from build123d import *

# Parameters (mm, degrees)
SALIENTE_EXTRUIR1_DEPTH = 10
CROQUIS2_R              = 3.5
SALIENTE_EXTRUIR2_DEPTH = 11
CROQUIS3_R              = 1
CORTAR_EXTRUIR1_DEPTH   = 40


with BuildPart() as part:
    # Croquis1 → Saliente-Extruir1 (new body)
    with BuildSketch(Plane(origin=(0, 0, 0), x_dir=(1, 0, 0), z_dir=(0, 1, 0))):
        Polygon((0, 6.639528096), (-5.75, 3.319764048), (-5.75, -3.319764048), (0, -6.639528096), (5.75, -3.319764048), (5.75, 3.319764048), align=None)
    extrude(amount=SALIENTE_EXTRUIR1_DEPTH)

    # Croquis2 → Saliente-Extruir2 (add)
    with BuildSketch(Plane.XZ):
        with Locations(Location((0, 0, 0), (0, 0, 270))):
            Circle(CROQUIS2_R)
    extrude(amount=SALIENTE_EXTRUIR2_DEPTH)

    # Croquis3 → Cortar-Extruir1 (cut)
    with BuildSketch(Plane.XZ.offset(11)):
        with Locations(Location((0, 0, 0), (0, 0, 270))):
            Circle(CROQUIS3_R)
    extrude(amount=-CORTAR_EXTRUIR1_DEPTH, mode=Mode.SUBTRACT)


solid = part.part
Part model, mm, in its own coordinate system. A direction names the side the tool comes from. Coordinates: 2 decimals unless noted, no trailing zeros. Write each loop counter-clockwise with the first axis right and the second up, starting at its lowest first coordinate (ties: lowest second). Pieces come first, ordered by that corner, then holes. Notation, with made-up numbers: M 79.5,-18 L 124.5,-18 A10 ccw 124.5,0 Z; hole C 77.25,69.5 d10. An arc over 180 degrees is marked long. Return JSON: item names as keys, results as strings.
1. 3-axis set-ups, long thin cutter, end or side, ignore diameter. For faces 4 (the face through (-3.417, -5.423, 0.759)), 5 (the face through (-0.1, 10, 1.4)): which of +Z, -Z, +X, -X, +Y, -Y reach the whole face in a straight line?
Determined:
{"face 4": "-Y", "face 5": "+Z, -Z, +X, -X, +Y"}
2. Pull direction Z, two halves, no side cores. Call faces 1 (the face through (-2.835, 4.93, -5.003)), 2 (the face through (-1, -1, 0)), 3 (the face through (-3, 0, 3)): pulls with the +Z half, pulls with the -Z half, needs draft (parallel to the pull), parting line crosses it, or undercut.
Determined:
{"face 1": "pulls with the -Z half", "face 2": "undercut", "face 3": "needs draft"}
3. Saw through at D-D, the plane z = 2.5. Write the cut outline in (x, y), then the cut area to 3 significant figures.
Determined:
{"outline": "M -5.75,0 L -2.45,0 L -2.45,-11 L 2.45,-11 L 2.45,0 L 5.75,0 L 5.75,10 L -5.75,10 Z", "area": "169 mm²"}
4. Saw through at A-A, the plane z = 0. Write the cut outline in (x, y).
Determined:
{"outline": "M -5.75,0 L -3.5,0 L -3.5,-11 L -1,-11 L -1,10 L -5.75,10 Z; M 1,-11 L 3.5,-11 L 3.5,0 L 5.75,0 L 5.75,10 L 1,10 Z"}
5. Saw through at B-B, the plane y = 5.5. Write the cut outline in (x, z), then the cut area to 3 significant figures.
Determined:
{"outline": "M -5.75,-3.32 L 0,-6.64 L 5.75,-3.32 L 5.75,3.32 L 0,6.64 L -5.75,3.32 Z; hole C 0,0 d2", "area": "111 mm²"}
6. Flat gauge pins, fed straight in: pin 1 Ø5 at (x, y) = (4, 3.5) entering from -Z; pin 2 Ø6 at (x, y) = (4.5, -8) entering from +Z. Where does each tip first touch, or does it go through?
Determined:
{"pin 1": "z = -5.77", "pin 2": "z = 3.16"}
7. Probe L1, parallel to X at y = -3.5, z = 0; L2, parallel to X at y = 5.25, z = 0; L3, parallel to Y at x = -0.25, z = 5.25. List the from-to ranges inside material, lowest first.
Determined:
{"L1": "-3.5 to -1, 1 to 3.5", "L2": "-5.75 to -1, 1 to 5.75", "L3": "0 to 10"}
8. Saw through at C-C, the plane x = 1.5. Write the cut outline in (y, z), then the cut area to 3 significant figures.
Determined:
{"outline": "M -11,-3.16 L 0,-3.16 L 0,-5.77 L 10,-5.77 L 10,5.77 L 0,5.77 L 0,3.16 L -11,3.16 Z", "area": "185 mm²"}
